Source: CAD feature listing. Evaluate the final solid. Frame: model axes, mm. Face numbers are marked on the shaded views. A direction names the side the tool comes from. Coordinates: 2 decimals unless noted, no trailing zeros. Loops run counter-clockwise (first coordinate to the right, second up) from the corner with the lowest first, then second, coordinate; pieces in that order, holes last. Notation, with made-up numbers: M 23,80.5 L 46,80.5 A23 cw 46,105.5 Z; hole C -39,41.5 d2. An arc over 180 degrees is marked long. One line per question, with ' | ' between items. Start each with the question number.
1. Pin query (flat end, axial travel): P1, Ø1, axis at x = 5, y = -1, coming from the +Z side; P2, Ø0.5, axis at x = 0.5, z = 0, coming from the -Y side. Return the tip coordinate at first contact, or that it passes through.
2. Access query for the marked faces 1 and 2. Directions: +Z, -Z, +X, -X, +Y, -Y. A direction counts if a zero-diameter tool reaches every point of the face in a straight line with its end or side. Return the directions, or none.
3. Section query A-A, the plane y = 0. Output: boundary loops of the cut face in (x, z).
4. Section query B-B, the plane z = 0. Output: boundary loops of the cut face in (x, y).
5. Ray query, probe 1 along Y at (x, z) = (6.5, 0.05); probe 2 along X at (y, z) = (0.95, 0.45); probe 3 along X at (y, z) = (-0.05, -1.25). Return the intervals inside material, ascending.
6. Section query C-C, the plane x = 4.75. Output: boundary loops of the cut face in (y, z), and give its area (3 significant figures).
```python
from build123d import *

# Parameters (mm, degrees)
FILLET2_R  = 0.1
SKETCH2_W  = 3
SKETCH2_H  = 0.4
SLOT_DEPTH = 0.45


with BuildPart() as part:
    # BodySke → Base-Revolve (revolve)
    with BuildSketch(Plane.XY):
        Polygon((1.1, 0.8), (1.1, 1.5), (0, 1.40376247), (0, 0), (9.1, 0), (9.1, 0.8), align=None)
    revolve(axis=Axis((-25.4, 0, 0), (1, 0, 0)))

    # Fillet2
    fillet2_edges = [part.edges().sort_by_distance(p)[0] for p in [
        (0, -1.40376247, 0),
    ]]
    fillet(fillet2_edges, radius=FILLET2_R)

    # Sketch2 → Slot (cut)
    with BuildSketch(Plane(origin=(0, 0, 0), x_dir=(0, 0, -1), z_dir=(1, 0, 0))):
        Rectangle(SKETCH2_W, SKETCH2_H)
    extrude(amount=SLOT_DEPTH, mode=Mode.SUBTRACT)


solid = part.part
```
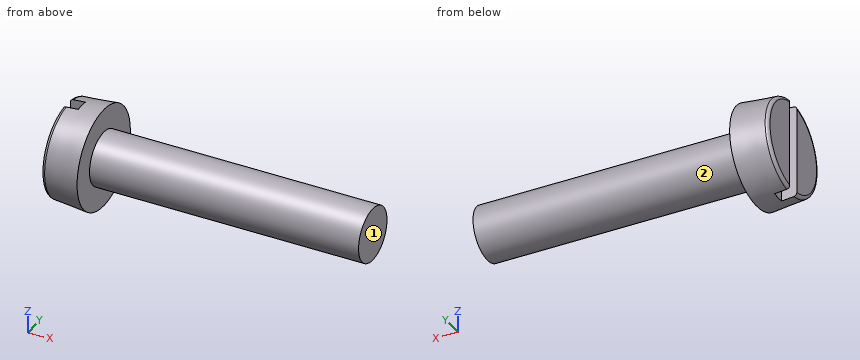
Taken from the geometry:
1) P1: z = 0.62 | P2: y = -1.47
2) face 1: +Z, -Z, +X, +Y, -Y | face 2: +X
3) outline: M 0.45,-1.44 L 1.1,-1.5 L 1.1,-0.8 L 9.1,-0.8 L 9.1,0.8 L 1.1,0.8 L 1.1,1.5 L 0.45,1.44 Z
4) outline: M 0,-1.31 A0.1 ccw 0.09,-1.41 L 1.1,-1.5 L 1.1,-0.8 L 9.1,-0.8 L 9.1,0.8 L 1.1,0.8 L 1.1,1.5 L 0.09,1.41 A0.1 ccw 0,1.31 L 0,0.2 L 0.45,0.2 L 0.45,-0.2 L 0,-0.2 Z
5) probe 1: -0.8 to 0.8 | probe 2: 0 to 1.1 | probe 3: 0.45 to 1.1
6) outline: C 0,0 d1.6 | area: 2.01 mm^2
